Read the model definition and answer for the solid it produces. Units are mm, in the model's axes. Face numbers are marked on the shaded views. Coordinates: 2 decimals unless noted, no trailing zeros. Loops run counter-clockwise (first coordinate to the right, second up) from the corner with the lowest first, then second, coordinate; pieces in that order, holes last.
Q1. Flat-ended cylindrical pins translate along their axes: P1, Ø2, axis at x = -1.5, y = -11, coming from the +Z side; P2, Ø5, axis at y = 3, z = 0, coming from the +X side (3 decimals); P3, Ø4, axis at y = 16, z = 5, coming from the -X side; P4, Ø1.5, axis at x = -2, z = 0, coming from the -Y side. Find the tip coordinate at first contact, or state that the pin passes through.
Q2. Section B-B (y = 19.5) is taken. Give the vertices of the cut face in (x, z).
Q3. Straight lines are drawn through the part: line 1 (X direction, y = 16.5, z = 0) (3 decimals); line 2 (Y direction, x = 0.5, z = -7.25); line 3 (Y direction, x = 6, z = -1). For each, find the intervals that lie inside material, in ascending order.
Q4. Section A-A (y = -10) is taken. Give the vertices of the cut face in (x, z) (3 decimals), then the cut area to 3 significant figures.
Q5. The mould has two halves that part along Z. Classify the marked faces 1, 2 and 3: pulls with the +Z half, pulls with the -Z half, needs draft (parallel to the pull), parting line crosses it, or undercut.
Autodesk Inventor part; units mm, degrees
ref_plane "YZ Plane" through (0, 0, 0) normal (1, 0, 0) x (0, 1, 0)
ref_plane "XZ Plane" through (0, 0, 0) normal (0, 1, 0) x (-1, 0, 0)
ref_plane "XY Plane" through (0, 0, 0) normal (0, 0, 1) x (1, 0, 0)
sketch "Sketch1" plane through (0, 0, 0) normal (1, 0, 0) x (0, 1, 0)
  line L0 (27.7812, 2.54) -> (0, 2.54)
  line L1 (-5.5563, 0) -> (33.3375, 0)
  line L2 (27.7812, 2.54) -> (27.7812, 7.9375)
  line L3 (0, 10.226) -> (0, -1.7043)
  line L4 (27.7812, 7.9375) -> (24.6063, 7.9375)
  line L5 (27.7812, 5.715) -> (0, 5.715)
  arc A0 (24.6063, 7.9375) -> (20.1613, 6.35) centre (24.6063, 0.9208) ccw
  arc A1 (18.3833, 5.715) -> (20.1613, 6.35) centre (18.3833, 8.5217) ccw
  point P0 (0, 0)
  dimension "d0" = 2.54
  dimension "d2" = 27.7812
  dimension "d3" = 3.175
  dimension "d5" = 3.175
  dimension "d6" = 7.62
  dimension "d9" = 7.9375
  dimension "d10" = 1.5875
revolve "Revolution1" add sketch "Sketch1" angle 360 about axis through (0, 0, 0) along (0, 1, 0)
mirror "Mirror1" about plane through (0, 0, 5.715) normal (0, -1, 0) of "Revolution1"
properties part number "Bolt_Spacer" material "ABS Plastic"
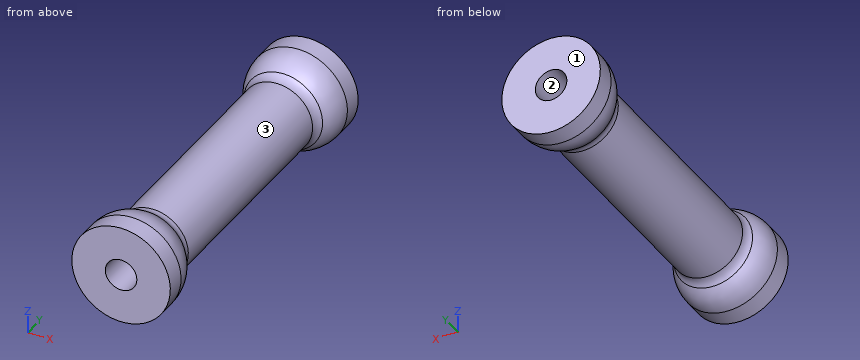
Numbers:
1. P1: stops at z = 5.69
1. P2: stops at x = 5.715
1. P3: stops at x = -4.86
1. P4: stops at y = -27.78
2. outline: circle Ø11.89 at (0, 0); hole circle Ø5.08 at (0, 0)
3. line 1: x = -5.715 to -2.54, 2.54 to 5.715
3. line 2: y = -27.78 to -21.61, 21.61 to 27.78
3. line 3: y = -27.78 to -19.77, 19.77 to 27.78
4. outline: circle Ø11.43 at (0, 0); hole circle Ø5.08 at (0, 0)
4. area: 82.3 mm2
5. face 1: needs draft
5. face 2: undercut
5. face 3: parting line crosses it
